Check sheet for the modelled part. Datum: model origin and axes. Units: mm. A direction names the side the tool comes from. Round coordinates to 2 decimals unless told otherwise and drop trailing zeros. Write each loop counter-clockwise with the first axis right and the second up, starting at its lowest first coordinate (ties: lowest second). Pieces come first, ordered by that corner, then holes. Notation, with made-up numbers: (-5, -4) - (24, -4) arc R27 ccw to (24, 24) - close; hole circle Ø3 at (76, 40). An arc over 180 degrees is marked (long way). Answer as a JSON object with one key per item and string values. Group by question number.
Item 1: Set-up check for faces 5 (the flat face through (2, -4, 0)), 6 (the flat face through (3, 0, 2.75)), 7 (the cylindrical face through (3.057, 3.009, 1.275)): record each of +Z, -Z, +X, -X, +Y, -Y from which the full face is reachable in a straight line by a thin tool's end or side.
Item 2: Sectioned sample at B-B on x = 3.75. Count the separate pieces of the cut face and the enclosed holes in it, plus the area to 3 significant figures.
Item 3: Thickness scan on line 1 (X direction, y = 0.25, z = -1); line 2 (Z direction, x = 4, y = 3.25); line 3 (Z direction, x = 2.75, y = -1) (3 decimals). Record the ranges inside material, lowest first.
Item 4: Sectioned sample at D-D on z = 3.5. Record the boundary of the cut face in (x, y).
Item 5: Release check for a two-part mould opening along X. For faces 1 (the flat face through (6.2, 0.1, 2.2)), 2 (the cylindrical face through (2.18, -0.06, -0.34)), 3 (the cylindrical face through (7.215, 0.056, -3.699)), 4 (the cylindrical face through (3.057, -2.991, 1.275)) record: pulls with the +X half, pulls with the -X half, needs draft (parallel to the pull), parting line crosses it, or undercut.
```python
from build123d import *

# Parameters (mm, degrees)
SKETCH1_W            = 8
SKETCH1_H            = 8
BOSS_EXTRUDE1_DEPTH  = 7.5
CUT_EXTRUDE1_DEPTH   = 6.2
M3_CLEARANCE_HOLE1_D = 3.4
FILLET1_R            = 1


with BuildPart() as part:
    # Sketch1 → Boss-Extrude1 (new body)
    with BuildSketch(Plane(origin=(0, 0, 0), x_dir=(0, 0, -1), z_dir=(1, 0, 0))):
        Rectangle(SKETCH1_W, SKETCH1_H)
    extrude(amount=BOSS_EXTRUDE1_DEPTH)

    # Sketch2 → Cut-Extrude1 (cut)
    with BuildSketch(Plane(origin=(0, 0, 0), x_dir=(0, 0, -1), z_dir=(1, 0, 0))):
        with BuildLine():
            Line((-2.025, 4), (-2.025, 3.740175425))
            ThreePointArc((-2.025, 3.740175425), (-1.987771412, 3.641268354), (-1.894565217, 3.591456891))
            ThreePointArc((-1.894565217, 3.591456891), (-1.736937846, 3.557611714), (-1.586797753, 3.498876404))
            ThreePointArc((-1.586797753, 3.498876404), (-1.275, 3), (-1.586797753, 2.501123596))
            ThreePointArc((-1.586797753, 2.501123596), (-1.736937846, 2.442388286), (-1.894565217, 2.408543109))
            ThreePointArc((-1.894565217, 2.408543109), (-1.987771412, 2.358731646), (-2.025, 2.259824575))
            Line((-2.025, 2.259824575), (-2.025, 2))
            Line((-2.025, 2), (-2.025, 1.740175425))
            ThreePointArc((-2.025, 1.740175425), (-1.987771412, 1.641268354), (-1.894565217, 1.591456891))
            ThreePointArc((-1.894565217, 1.591456891), (-1.736937846, 1.557611714), (-1.586797753, 1.498876404))
            ThreePointArc((-1.586797753, 1.498876404), (-1.275, 1), (-1.586797753, 0.501123596))
            ThreePointArc((-1.586797753, 0.501123596), (-1.736937846, 0.442388286), (-1.894565217, 0.408543109))
            ThreePointArc((-1.894565217, 0.408543109), (-1.987771412, 0.358731646), (-2.025, 0.259824575))
            Line((-2.025, 0.259824575), (-2.025, 0))
            Line((-2.025, 0), (-2.025, -0.259824575))
            ThreePointArc((-2.025, -0.259824575), (-1.987771412, -0.358731646), (-1.894565217, -0.408543109))
            ThreePointArc((-1.894565217, -0.408543109), (-1.736937846, -0.442388286), (-1.586797753, -0.501123596))
            ThreePointArc((-1.586797753, -0.501123596), (-1.275, -1), (-1.586797753, -1.498876404))
            ThreePointArc((-1.586797753, -1.498876404), (-1.736937846, -1.557611714), (-1.894565217, -1.591456891))
            ThreePointArc((-1.894565217, -1.591456891), (-1.987771412, -1.641268354), (-2.025, -1.740175425))
            Line((-2.025, -1.740175425), (-2.025, -2))
            Line((-2.025, -2), (-2.025, -2.259824575))
            ThreePointArc((-2.025, -2.259824575), (-1.987771412, -2.358731646), (-1.894565217, -2.408543109))
            ThreePointArc((-1.894565217, -2.408543109), (-1.736937846, -2.442388286), (-1.586797753, -2.501123596))
            ThreePointArc((-1.586797753, -2.501123596), (-1.275, -3), (-1.586797753, -3.498876404))
            ThreePointArc((-1.586797753, -3.498876404), (-1.736937846, -3.557611714), (-1.894565217, -3.591456891))
            ThreePointArc((-1.894565217, -3.591456891), (-1.987771412, -3.641268354), (-2.025, -3.740175425))
            Line((-2.025, -3.740175425), (-2.025, -4))
            Line((-2.025, -4), (-2.75, -4))
            Line((-2.75, -4), (-2.75, 4))
            Line((-2.75, 4), (-2.025, 4))
        make_face()
    extrude(amount=CUT_EXTRUDE1_DEPTH, mode=Mode.SUBTRACT)

    # M3 Clearance Hole1 (through all)
    with Locations(Plane(origin=(0, 4, 0), x_dir=(1, 0, 0), z_dir=(0, 1, 0))):
        with Locations((3.75, 0.9875)):
            Hole(M3_CLEARANCE_HOLE1_D / 2)

    # Fillet1
    fillet1_edges = [part.edges().sort_by_distance(p)[0] for p in [
        (7.5, 0, 4),
        (7.5, 0, -4),
        (0, 0, 4),
        (0, 0, -4),
        (3.75, -4, 4),
    ]]
    fillet(fillet1_edges, radius=FILLET1_R)


solid = part.part
```
Completed:
{
 "1": {"face 5": "+Z, -Z, +X, -X, -Y", "face 6": "-X, +Y, -Y", "face 7": "-X"},
 "2": {"separate pieces": "3", "enclosed holes": "0", "area": "27.9 mm²"},
 "3": {"line 1": "0 to 2.05, 5.45 to 7.5", "line 2": "-4 to -2.67, 0.69 to 1.33, 2.75 to 4", "line 3": "-4 to -2.362, 0.387 to 1.275, 2.75 to 4"},
 "4": {"outline": "(0.13, -3.87) - (7.37, -3.87) - (7.37, 4) - (0.13, 4) - close"},
 "5": {"face 1": "pulls with the -X half", "face 2": "undercut", "face 3": "pulls with the +X half", "face 4": "needs draft"}
}
